from build123d import *

# Parameters (mm, degrees)
F0_R     = 7.9375
F1_DEPTH = 12.7


with BuildPart() as f1:
    # F0 (on Front) → F1 (new body)
    with BuildSketch(Plane.XZ):
        with BuildLine():
            Line((-33.147, -33.147), (0, 0))
            Line((0, 0), (-13.843, 13.843))
            Line((-13.843, 13.843), (-112.556101, 13.843))
            Line((-112.556101, 13.843), (-151.850627, -19.129022))
            ThreePointArc((-151.850627, -19.129022), (-154.20731, -27.924285), (-146.7485, -33.147))
            Line((-146.7485, -33.147), (-33.147, -33.147))
        make_face()
        with Locations((-102.87, -9.652)):
            Circle(F0_R, mode=Mode.SUBTRACT)
        with Locations((-80.645, -9.652)):
            Circle(F0_R, mode=Mode.SUBTRACT)
        with Locations((-58.42, -9.652)):
            Circle(F0_R, mode=Mode.SUBTRACT)
    extrude(amount=F1_DEPTH)


solid = f1.part
Verification items for the finished model (mm, model axes). Give positions to 0.01 mm unless a question says otherwise; leave off trailing zeros. Write each loop counter-clockwise with the first axis right and the second up, starting at its lowest first coordinate (ties: lowest second). Pieces come first, ordered by that corner, then holes.
(1) Mould release check, pull along Z, two halves, no side actions. Record for faces 1 (the face through (-50.85, -6.26, -7.27)), 2 (the face through (-73.074, -6.261, -7.268)), 3 (the face through (-78, -12.7, -20)), 4 (the face through (-63, -6, 13.843)): +Z half, -Z half, draft (parallel to the pull), parting line (faces both ways), or undercut.
(2) Cross-section at C-C (x = -136). Enter the section's corners in (y, z).
(3) Material ranges on line 1 (Z direction, x = -58.42, y = -5.5); line 2 (X direction, y = -7, z = -7.5); line 3 (X direction, y = -3, z = -8), recorded low to high.
(4) Cross-section at A-A (x = -102.87). Enter the section's corners in (y, z).
(5) Cross-section at B-B (y = -2). Enter the section's corners in (x, z) (1 decimal).
(6) Gauge pin test, flat ends, axial feed: pin 1 (3 mm diameter, centred on y = -4.5, z = -7.5, fed in from +X); pin 2 (1 mm diameter, centred on y = -8.5, z = -26.5, fed in from +X); pin 3 (2 mm diameter, centred on y = -10, z = 9, fed in from +X). Record the tip position at first contact, or that the pin passes through.
Worked out:
1. face 1: undercut
1. face 2: undercut
1. face 3: draft
1. face 4: +Z half
2. outline: (-12.7, -33.15) - (0, -33.15) - (0, -5.83) - (-12.7, -5.83) - close
3. line 1: z = -33.15 to -17.59, -1.71 to 13.84
3. line 2: x = -137.99 to -110.51, -95.23 to -88.29, -73 to -66.06, -50.78 to -7.5
3. line 3: x = -138.59 to -110.63, -95.11 to -88.41, -72.88 to -66.18, -50.66 to -8
4. outline: (-12.7, -33.15) - (0, -33.15) - (0, -17.59) - (-12.7, -17.59) - close; (-12.7, -1.71) - (0, -1.71) - (0, 13.84) - (-12.7, 13.84) - close
5. outline: (-151.9, -19.1) arc R7.9 ccw to (-146.7, -33.1) - (-33.1, -33.1) - (0, 0) - (-13.8, 13.8) - (-112.6, 13.8) - close; hole circle Ø15.9 at (-102.9, -9.7); hole circle Ø15.9 at (-80.6, -9.7); hole circle Ø15.9 at (-58.4, -9.7)
6. pin 1: stops at x = -6
6. pin 2: stops at x = -26
6. pin 3: stops at x = -8
